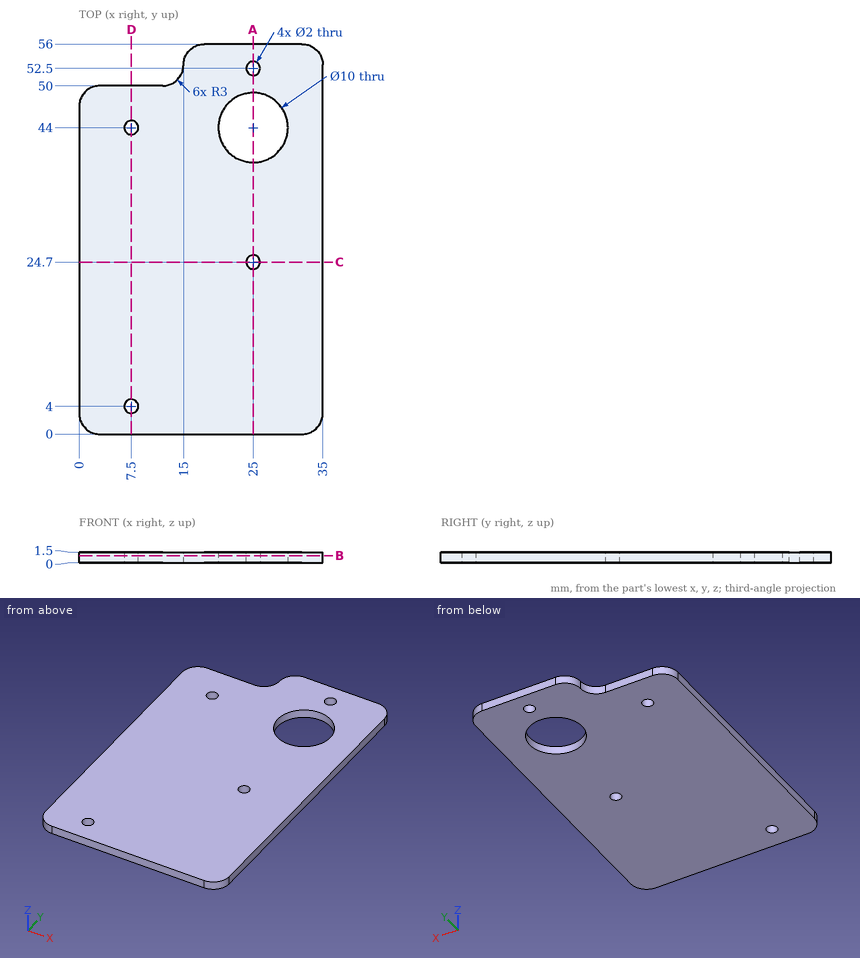
Here's the drawing with two shaded views (mm, measured from the low corner). I have some questions. Coordinates: 2 decimals unless noted, no trailing zeros. Order: outer loops, then holes, each group sorted by start corner. A loop starts at its lowest first (then second) coordinate and runs counter-clockwise, first axis right, second up.
Q1. Suppose I cut it at C-C on y = 24.7. Please give me the cut outline in (x, z), and give its area (3 significant figures).
Q2. Suppose I cut it at A-A on x = 25. Please give me the cut outline in (y, z), and give its area (3 significant figures).
Q3. Suppose I cut it at D-D on x = 7.5. Please give me the cut outline in (y, z), and give its area (3 significant figures).
Q4. Suppose I cut it at B-B on z = 1. Give the number of separate pieces and of enclosed holes in the cut face, and give its area (3 significant figures).
Q5. Please list where these lines run through material, in increasing order: L1, parallel to Y at x = 7.5, z = 0.5; L2, parallel to X at y = 4.5, z = 0.95; L3, parallel to X at y = 43.5, z = 0.45 (1 decimal).
Answer:
1. outline: (0, 0) - (24, 0) - (24, 1.5) - (0, 1.5) - close; (26, 0) - (35, 0) - (35, 1.5) - (26, 1.5) - close
1. area: 49.5 mm2
2. outline: (0, 0) - (23.7, 0) - (23.7, 1.5) - (0, 1.5) - close; (25.7, 0) - (39, 0) - (39, 1.5) - (25.7, 1.5) - close; (49, 0) - (51.5, 0) - (51.5, 1.5) - (49, 1.5) - close; (53.5, 0) - (56, 0) - (56, 1.5) - (53.5, 1.5) - close
2. area: 63.0 mm2
3. outline: (0, 0) - (3, 0) - (3, 1.5) - (0, 1.5) - close; (5, 0) - (43, 0) - (43, 1.5) - (5, 1.5) - close; (45, 0) - (50, 0) - (50, 1.5) - (45, 1.5) - close
3. area: 69.0 mm2
4. separate pieces: 1
4. enclosed holes: 5
4. area: 1,770 mm2
5. L1: y = 0 to 3, 5 to 43, 45 to 50
5. L2: x = 0 to 6.63, 8.37 to 35
5. L3: x = 0 to 6.6, 8.4 to 20, 30 to 35
